from build123d import *

# Parameters (mm, degrees)
SKETCH_W     = 5.34
SKETCH_H     = 136
PAD_DEPTH    = 4
PAD001_DEPTH = 5.34
SKETCH002_W  = 10
SKETCH002_H  = 14
SKETCH002_R  = 1.65
PAD002_DEPTH = 4
FILLET_R     = 2
FILLET001_R  = 1.99


with BuildPart() as part:
    # Sketch → Pad (new body)
    with BuildSketch(Plane.XY):
        with Locations((-2.67, 0)):
            Rectangle(SKETCH_W, SKETCH_H)
    extrude(amount=-PAD_DEPTH)

    # Sketch001 → Pad001 (join)
    with BuildSketch(Plane.YZ):
        with BuildLine():
            ThreePointArc((59.287408, 0), (55.84916, 22.338654), (45.852682, 42.609507))
            Line((45.852682, 42.609507), (28.071813, 68.00322))
            Line((26.92466, 69.641524), (28.071813, 68.00322))
            Line((22.828899, 66.773642), (26.92466, 69.641524))
            Line((23.976052, 65.135338), (22.828899, 66.773642))
            Line((24.795204, 65.708914), (23.976052, 65.135338))
            Line((24.795204, 65.708914), (40.281768, 43.591809))
            Line((40.281768, 43.591809), (-21.973787, 0))
            Line((-21.973787, 0), (-37.460351, 22.117105))
            Line((-36.641199, 22.690682), (-37.460351, 22.117105))
            Line((-37.788352, 24.328986), (-36.641199, 22.690682))
            Line((-41.884112, 21.461104), (-37.788352, 24.328986))
            Line((-40.736959, 19.822799), (-41.884112, 21.461104))
            Line((-40.736959, 19.822799), (-26.856886, 0))
            Line((-26.856886, 0), (-26.856886, -1))
            Line((-26.856886, -1), (-15, -1))
            Line((-15, -1), (-15, 0))
            Line((-15, 0), (42.576074, 40.315201))
            ThreePointArc((55.287408, 0), (52.034292, 21.135831), (42.576074, 40.315201))
            Line((55.287408, 0), (59.287408, 0))
        make_face()
    extrude(amount=-PAD001_DEPTH)

    # Sketch002 → Pad002 (join)
    with BuildSketch(Plane.XY):
        with Locations((5, 61)):
            Rectangle(SKETCH002_W, SKETCH002_H)
        with Locations((5, 60)):
            Circle(SKETCH002_R, mode=Mode.SUBTRACT)
        with Locations((5, -61)):
            Rectangle(SKETCH002_W, SKETCH002_H)
        with Locations((5, -60)):
            Circle(SKETCH002_R, mode=Mode.SUBTRACT)
    extrude(amount=-PAD002_DEPTH)

    # Fillet
    fillet_edges = [part.edges().sort_by_distance(p)[0] for p in [
        (10, 61, 0),
        (10, -61, 0),
        (5, -68, 0),
        (5, 68, 0),
        (-2.67, -26.856886, 0),
        (-2.67, -15, 0),
        (-2.67, 42.576074, 40.315201),
    ]]
    fillet(fillet_edges, radius=FILLET_R)

    # Fillet001
    fillet001_edges = [part.edges().sort_by_distance(p)[0] for p in [
        (5, -68, -4),
        (5, 68, -4),
        (5, 54, -4),
        (5, -54, -4),
        (-2.67, -41.884112, 21.461104),
        (-2.67, 26.92466, 69.641524),
    ]]
    fillet(fillet001_edges, radius=FILLET001_R)


solid = part.part
Check sheet for the modelled part. Datum: model origin and axes. Units: mm. A direction names the side the tool comes from. Give positions to 0.01 mm unless a question says otherwise; leave off trailing zeros. Order: outer loops, then holes, each group sorted by start corner. A loop starts at its lowest first (then second) coordinate and runs counter-clockwise, first axis right, second up. Notation, with made-up numbers: M 85,58.5 L 115,58.5 A31 ccw 115,93.5 Z; hole C 1.5,12 d11. An arc over 180 degrees is marked long. Answer as CSV lines item,"result". Start each with the question number.
Item 1: Gauge pin test, flat ends, axial feed: P1, Ø2, axis at x = 3, z = -0.5, coming from the +Y side; P2, Ø6, axis at x = -1, y = 42.5, coming from the +Z side; P3, Ø3, axis at y = -0.5, z = 13, coming from the +X side. Record the tip position at first contact, or that the pin passes through.
Item 2: Cross-section at C-C on y = -60. Enter the section's corners in (x, z), plus the area to 3 significant figures.
Item 3: Cross-section at B-B on z = 30.5. Enter the section's corners in (x, y), plus the area to 3 significant figures.
Item 4: Tool access check on faces 1 (the face through (-2.707, 26.803, 68.826)), 2 (the face through (-0.2, -52, 0)), 3 (the face through (-2.633, 52.418, 19.878)). Record the directions out of +Z, -Z, +X, -X, +Y, -Y that give a thin tool (end or side, any length) a straight path to the whole face; none if there is none.
Item 5: Mould release check, pull along Z, two halves, no side actions. Record for faces 4 (the face through (-5.34, 10, 19)), 5 (the face through (-2.707, -41.076, 21.296)), 6 (the face through (-2.633, -39.038, 23.454)): +Z half, -Z half, draft (parallel to the pull), parting line (faces both ways), or undercut.
Item 6: Thickness scan on line 1 (Y direction, x = 5, z = -2.1); line 2 (Y direction, x = -0.75, z = 9.5); line 3 (Y direction, x = 5, z = -1.2). Record the ranges inside material, lowest first. Write a range as [from, to].
Item 7: Cross-section at A-A on x = 5. State how many separate pieces and enclosed holes the cut face has, plus the area to 3 significant figures.
Item 8: Cross-section at D-D on z = 6. Enter the section's corners in (x, y), plus the area to 4 significant figures.
Established:
1,P1,"stops at y = 67.94"
1,P2,"stops at z = 51.68"
1,P3,"stops at x = 0"
2,outline,"M -5.34,-4 L 3.35,-4 L 3.35,0 L -5.34,0 Z; M 6.65,-4 L 10,-4 L 10,-2 A2 ccw 8,0 L 6.65,0 Z"
2,area,"47.3 mm^2"
3,outline,"M -5.34,21.58 L 0,21.58 L 0,28.56 L -5.34,28.56 Z; M -5.34,48.33 L 0,48.33 L 0,52.74 L -5.34,52.74 Z"
3,area,"60.8 mm^2"
4,face 1,"+Z, +X, -X"
4,face 2,"+X, -X, -Y"
4,face 3,"+X, -X"
5,face 4,"draft"
5,face 5,"undercut"
5,face 6,"+Z half"
6,line 1,"y = [-68, -61.65], [-58.35, -54], [54, 58.35], [61.65, 68]"
6,line 2,"y = [-33.51, -28.63], [-8.41, -1.43], [54.64, 58.68]"
6,line 3,"y = [-67.83, -61.65], [-58.35, -54], [54, 58.35], [61.65, 67.83]"
7,separate pieces,"4"
7,enclosed holes,"0"
7,area,"80.5 mm^2"
8,outline,"M -5.34,-31.06 L 0,-31.06 L 0,-26.18 L -5.34,-26.18 Z; M -5.34,-13.4 L 0,-13.4 L 0,-6.43 L -5.34,-6.43 Z; M -5.34,55.03 L 0,55.03 L 0,59.04 L -5.34,59.04 Z"
8,area,"84.75 mm^2"
